Work out the finished part from the listing and answer in its coordinate system (mm). Give positions to 0.01 mm unless a question says otherwise; leave off trailing zeros. Loops run counter-clockwise (first coordinate to the right, second up) from the corner with the lowest first, then second, coordinate; pieces in that order, holes last. Notation, with made-up numbers: (7, -5.5) -> (44, -5.5) arc R18 cw to (44, 1.5) -> close; hole circle Ø2 at (-14.5, 35.5). An arc over 180 degrees is marked (long way). Answer as CSV lines item,"result". Start each with the question number.
1. Find section B-B, the plane y = -17.2. Give the vertices of the cut face in (x, z) (3 decimals).
2. Find section C-C, the plane z = 5. Give the vertices of the cut face in (x, y).
3. Find the intervals of material crossed by line 1 along Z through (x, y) = (-32.5, -17.4); line 2 along Z through (x, y) = (-31.25, -17.05); line 3 along X through (y, z) = (-16.95, 3), in increasing order.
4. Flat-ended cylindrical pins translate along their axes: pin 1 Ø1.9 at (x, z) = (-13.21, -2.74) entering from +Y; pin 2 Ø1 at (y, z) = (-17, 19) entering from +X; pin 3 Ø1.6 at (y, z) = (-17.5, 14.5) entering from -X. Find the tip coordinate at first contact, or state that the pin passes through.
5. Find section A-A, the plane x = -12.5. Give the vertices of the cut face in (y, z), and give its area (3 significant figures).
6. Find section D-D, the plane x = -23.75. Give the vertices of the cut face in (y, z).
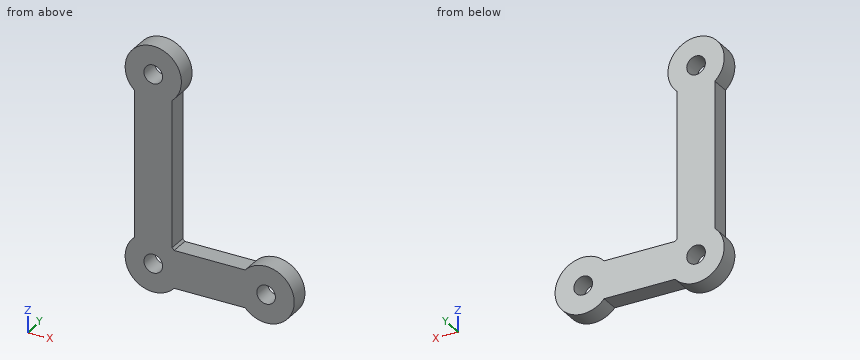
from build123d import *

# Parameters (mm, degrees)
LIFT_ARM_START         = -18.881702924
LIFT_ARM_OUTLINE_R     = 1.575
LIFT_ARM_DEPTH         = 3.175
LIFT_ARM_SKETCH_R      = 1.575
LIFT_ARM_EXTRUDE_DEPTH = 3.175


# Read off the part's stored shape, not the designer's step: Lift_Arm
with BuildPart() as part:
    # Lift_Arm outline → Lift_Arm (new body)
    with BuildSketch(Plane(origin=(0, 0, 0), x_dir=(1, 0, 0), z_dir=(0, 1, 0)).offset(LIFT_ARM_START)):
        with BuildLine():
            ThreePointArc((-35.433976258, -25.480614034), (-32.258976258, -33.763583748), (-29.083976258, -25.480614034))
            Line((-29.083976258, -25.480614034), (-29.083976258, -0.796553462))
            ThreePointArc((-29.083976258, -0.796553462), (-32.258976258, 7.486416252), (-35.433976258, -0.796553462))
            Line((-35.433976258, -0.796553462), (-35.433976258, -25.480614034))
        make_face()
        with Locations((-32.258976258, -29.013583748)):
            Circle(LIFT_ARM_OUTLINE_R, mode=Mode.SUBTRACT)
        with Locations((-32.258976258, 2.736416252)):
            Circle(LIFT_ARM_OUTLINE_R, mode=Mode.SUBTRACT)
    extrude(amount=LIFT_ARM_DEPTH)

    # Lift Arm Sketch → Lift Arm Extrude (add)
    with BuildSketch(Plane.XZ.offset(18.881702924)):
        with BuildLine():
            ThreePointArc((-28.726006544, 0.438583748), (-27.508976258, -2.736416252), (-28.726006544, -5.911416252))
            Line((-28.726006544, -5.911416252), (-16.741945972, -5.911416252))
            ThreePointArc((-16.741945972, -5.911416252), (-8.458976258, -2.736416252), (-16.741945972, 0.438583748))
            Line((-16.741945972, 0.438583748), (-28.726006544, 0.438583748))
        make_face()
        with Locations(Location((-13.208976258, -2.736416252, 0), (0, 0, 270))):
            Circle(LIFT_ARM_SKETCH_R, mode=Mode.SUBTRACT)
    extrude(amount=-LIFT_ARM_EXTRUDE_DEPTH)


solid = part.part
Resolved:
1,outline,"(-35.434, 0.797) arc R4.75 ccw (long way) to (-28.726, -5.911) -> (-16.742, -5.911) arc R4.75 ccw (long way) to (-16.742, 0.439) -> (-28.726, 0.439) arc R4.75 ccw to (-29.084, 0.797) -> (-29.084, 25.481) arc R4.75 ccw (long way) to (-35.434, 25.481) -> close; hole circle Ø3.15 at (-32.259, -2.736); hole circle Ø3.15 at (-32.259, 29.014); hole circle Ø3.15 at (-13.209, -2.736)"
2,outline,"(-35.43, -18.88) -> (-29.08, -18.88) -> (-29.08, -15.71) -> (-35.43, -15.71) -> close"
3,line 1,"z = -7.48 to -4.29, -1.18 to 27.46, 30.57 to 33.76"
3,line 2,"z = -7.38 to -3.95, -1.53 to 27.8, 30.22 to 33.66"
3,line 3,"x = -35.43 to -29.08"
4,pin 1,"passes through"
4,pin 2,"stops at x = -29.08"
4,pin 3,"stops at x = -35.43"
5,outline,"(-18.88, -7.43) -> (-15.71, -7.43) -> (-15.71, -4.14) -> (-18.88, -4.14) -> close; (-18.88, -1.33) -> (-15.71, -1.33) -> (-15.71, 1.96) -> (-18.88, 1.96) -> close"
5,area,"20.9 mm^2"
6,outline,"(-18.88, -5.91) -> (-15.71, -5.91) -> (-15.71, 0.44) -> (-18.88, 0.44) -> close"
